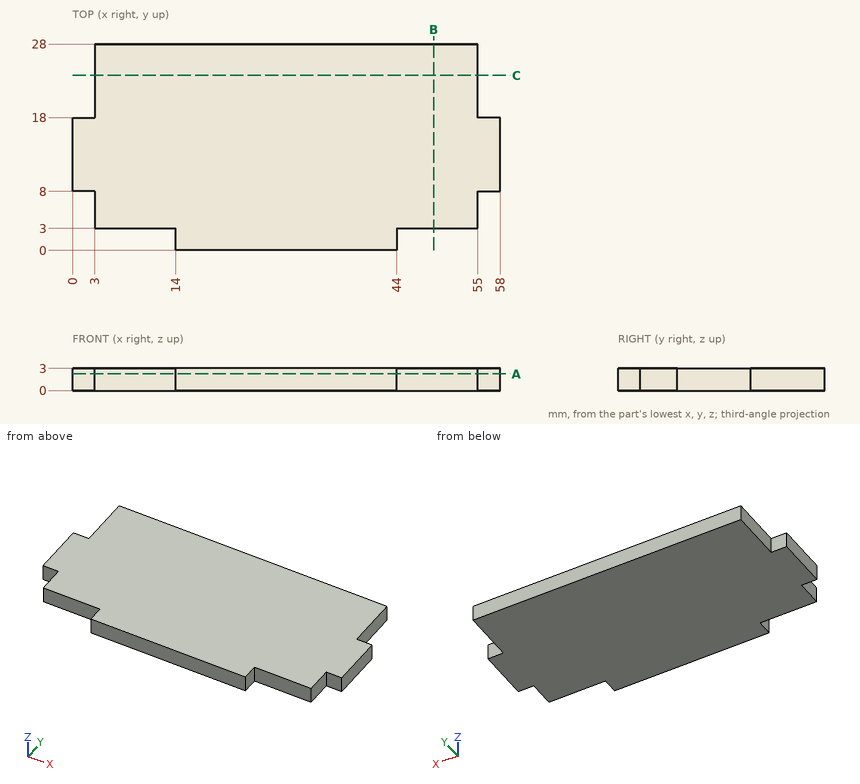
Answer from the drawing. Dimensions are ordinates in mm from the lowest x, y and z of the part. Coordinates: 2 decimals unless noted, no trailing zeros. Loops run counter-clockwise (first coordinate to the right, second up) from the corner with the lowest first, then second, coordinate; pieces in that order, holes last.
Q1. Consider probe 1 along Y at (x, z) = (12.5, 1.25); probe 2 along X at (y, z) = (19.5, 2.3); probe 3 along Y at (x, z) = (55.5, 0.45). Determine where each line is inside the solid, lowest interval first.
Q2. Each of these flat-tipped pins is pushed along its axis until it touches: pin 1 Ø0.9 at (x, z) = (1, 1) entering from +Y; pin 2 Ø0.9 at (y, z) = (5.5, 1) entering from -X; pin 3 Ø0.9 at (x, z) = (56, 1.5) entering from -Y. Where does it stop, or does it pass through?
Q3. The part is cut by section C-C on y = 23.75. Write down the section's boundary in (x, z).
Q4. The part is cut by section B-B on x = 49. Write down the section's boundary in (y, z).
Q5. The part is cut by section A-A on z = 2.25. Write down the section's boundary in (x, y), and give its area (3 significant figures).
Results below:
1. probe 1: y = 3 to 28
1. probe 2: x = 3 to 55
1. probe 3: y = 8 to 18
2. pin 1: stops at y = 18
2. pin 2: stops at x = 3
2. pin 3: stops at y = 8
3. outline: (3, 0) - (55, 0) - (55, 3) - (3, 3) - close
4. outline: (3, 0) - (28, 0) - (28, 3) - (3, 3) - close
5. outline: (0, 8) - (3, 8) - (3, 3) - (14, 3) - (14, 0) - (44, 0) - (44, 3) - (55, 3) - (55, 8) - (58, 8) - (58, 18) - (55, 18) - (55, 28) - (3, 28) - (3, 18) - (0, 18) - close
5. area: 1,450 mm2
